Can you work these out from the model? Positions are in its coordinate system, mm. A direction names the side the tool comes from. Give positions to 0.01 mm unless a question says otherwise; leave off trailing zeros. Order: outer loops, then holes, each group sorted by start corner. A loop starts at its lowest first (then second) coordinate and runs counter-clockwise, first axis right, second up. Notation, with made-up numbers: (-37, 82.5) - (-9, 82.5) arc R11 ccw to (-9, 87.5) - close; hole circle Ø1 at (56, 57). An arc over 180 degrees is marked (long way). Answer as a JSON object with one key per item and string values.
```python
from build123d import *

# Parameters (mm, degrees)
SKETCH1_R                        = 6.35
BOSS_EXTRUDE1_DEPTH              = 3.175
SKETCH2_R                        = 4.699
BOSS_EXTRUDE2_DEPTH              = 143.256
F_97_0_0059_DIAMETER_HOLE1_D     = 6.35
F_97_0_0059_DIAMETER_HOLE1_DEPTH = 143.256


with BuildPart() as part:
    # Sketch1 → Boss-Extrude1 (new body)
    with BuildSketch(Plane(origin=(0, 0, 0), x_dir=(1, 0, 0), z_dir=(0, 1, 0))):
        with Locations(Location((0, 0, 0), (0, 0, 270))):
            Circle(SKETCH1_R)
    extrude(amount=-BOSS_EXTRUDE1_DEPTH)

    # Sketch2 → Boss-Extrude2 (add)
    with BuildSketch(Plane(origin=(0, 0, 0), x_dir=(1, 0, 0), z_dir=(0, 1, 0))):
        with Locations(Location((0, 0, 0), (0, 0, 270))):
            Circle(SKETCH2_R)
    extrude(amount=BOSS_EXTRUDE2_DEPTH)

    # #97 (0.0059) Diameter Hole1
    with Locations(Plane(origin=(0, -3.175, 0), x_dir=(0, 0, -1), z_dir=(0, -1, 0))):
        with Locations((0, 0)):
            Hole(F_97_0_0059_DIAMETER_HOLE1_D / 2, depth=F_97_0_0059_DIAMETER_HOLE1_DEPTH)


solid = part.part
```
Q1. We'd pull the mould along Z, two halves only. Please class faces 1 (the face through (0, 140.081, 0)), 2 (the face through (-3.1, 69.46, -0.69)), 3 (the face through (4.66, 70.63, -0.61)), 4 (the face through (0, 143.256, 0)): released by +Z, released by -Z, zero draft, split by the parting line, or undercut.
Recorded:
{"face 1": "undercut", "face 2": "undercut", "face 3": "split by the parting line", "face 4": "zero draft"}
Q2. Which directions (+Z, -Z, +X, -X, +Y, -Y) give clear straight access to the entire face, cutting with the end or side of a thin tool? Please do faces 5 (the face through (-3.86, -1.57, -5.04)), 6 (the face through (5, 0, 0)).
Recorded:
{"face 5": "+Y, -Y", "face 6": "+Y"}
Q3. If we section it at C-C, the plane y = 72: Please give me the cut outline in (x, z) (3 decimals), then the cut area to 3 significant figures.
Recorded:
{"outline": "circle Ø9.398 at (0, 0); hole circle Ø6.35 at (0, 0)", "area": "37.7 mm^2"}
Q4. I need wall thicknesses on L1, parallel to X at y = 57, z = 0 (3 decimals); L2, parallel to X at y = 82.5, z = 0.5; L3, parallel to Y at x = 5.75, z = -0.25 (3 decimals). Which ranges of each line are inside material? Lowest first, please.
Recorded:
{"L1": "x = -4.699 to -3.175, 3.175 to 4.699", "L2": "x = -4.67 to -3.14, 3.14 to 4.67", "L3": "y = -3.175 to 0"}
Q5. If we section it at B-B, the plane x = 0: Please give me the cut outline in (y, z) (3 decimals).
Recorded:
{"outline": "(-3.175, -6.35) - (0, -6.35) - (0, -4.699) - (143.256, -4.699) - (143.256, 4.699) - (0, 4.699) - (0, 6.35) - (-3.175, 6.35) - (-3.175, 3.175) - (140.081, 3.175) - (140.081, -3.175) - (-3.175, -3.175) - close"}
Q6. If we section it at A-A, the plane z = 0: Please give me the cut outline in (x, y) (3 decimals).
Recorded:
{"outline": "(-6.35, -3.175) - (-3.175, -3.175) - (-3.175, 140.081) - (3.175, 140.081) - (3.175, -3.175) - (6.35, -3.175) - (6.35, 0) - (4.699, 0) - (4.699, 143.256) - (-4.699, 143.256) - (-4.699, 0) - (-6.35, 0) - close"}
Q7. I'm going to push flat-ended pins straight in: pin 1 Ø2 at (x, y) = (3.5, 46.5) entering from -Z; pin 2 Ø1 at (y, z) = (39, -4) entering from -X; pin 3 Ø6 at (y, z) = (32, -3) entering from +X. Where does each tip first touch, or does it pass through?
Recorded:
{"pin 1": "stops at z = -3.98", "pin 2": "stops at x = -3.14", "pin 3": "stops at x = 4.7"}
